The model under review builds one solid part; all positions refer to its coordinate system, in mm. Round coordinates to 2 decimals unless told otherwise and drop trailing zeros.
```python
from build123d import *

# Parameters (mm, degrees)
BOSS_EXTRUDE1_DEPTH   = 4.7625
M3_CLEARANCE_HOLE1_D  = 3.4
F_8_CLEARANCE_HOLE1_D = 4.4958
CIRPATTERN1_COUNT     = 12
CUT_EXTRUDE1_REACH    = 272.048
SKETCH15_W            = 6.35
SKETCH15_H            = 62.484
SKETCH15_W_2          = 5.116657908
SKETCH15_H_2          = 18.000886741
SKETCH15_H_3          = 20.68418835
SKETCH15_W_3          = 7.62
CUT_EXTRUDE2_REACH    = 272.048
SKETCH17_R            = 2.2479


with BuildPart() as part:
    # Sketch1 → Boss-Extrude1 (new body)
    with BuildSketch(Plane(origin=(0, 0, 0), x_dir=(1, 0, 0), z_dir=(0, 1, 0))):
        with BuildLine():
            Line((177.8, 98.373776994), (177.8, -98.373776994))
            ThreePointArc((177.8, -98.373776994), (0, -203.2), (-177.8, -98.373776994))
            Line((-177.8, -98.373776994), (-177.8, 98.373776994))
            ThreePointArc((-177.8, 98.373776994), (0, 203.2), (177.8, 98.373776994))
        make_face()
    extrude(amount=BOSS_EXTRUDE1_DEPTH)

    # M3 Clearance Hole1 (through all)
    with Locations(Plane(origin=(0, 4.7625, 0), x_dir=(1, 0, 0), z_dir=(0, 1, 0))):
        with Locations((174.55, -94.8), (174.55, -80), (174.55, -65.2), (174.55, 65.2), (174.55, 80), (174.55, 94.8)):
            m3_clearance_hole1 = Hole(M3_CLEARANCE_HOLE1_D / 2)

    # Mirror1: M3 Clearance Hole1 across plane
    add(m3_clearance_hole1.mirror(Plane(origin=(0, 0, 0), x_dir=(0, 0, 1), z_dir=(1, 0, 0))), mode=Mode.SUBTRACT)

    # #8 Clearance Hole1 (through all)
    with Locations(Plane(origin=(0, 4.7625, 0), x_dir=(1, 0, 0), z_dir=(0, 1, 0))):
        with Locations((0, -142.875)):
            f_8_clearance_hole1 = Hole(F_8_CLEARANCE_HOLE1_D / 2)

    # CirPattern1: #8 Clearance Hole1 ×12 about axis
    cirpattern1_axis = Axis((0, 0, 0), (0, 1, 0))
    for i in range(1, CIRPATTERN1_COUNT):
        add(f_8_clearance_hole1.rotate(cirpattern1_axis, i * 360 / CIRPATTERN1_COUNT), mode=Mode.SUBTRACT)

    # Sketch15 → Cut-Extrude1 (cut, up to next)
    with BuildSketch(Plane(origin=(0, 4.7625, 0), x_dir=(1, 0, 0), z_dir=(0, 1, 0)), mode=Mode.PRIVATE) as cut_extrude1_sk1:
        with Locations((24.765, 31.242)):
            Rectangle(SKETCH15_W, SKETCH15_H)
    cut_extrude1_tool1 = extrude(cut_extrude1_sk1.sketch, amount=-CUT_EXTRUDE1_REACH, mode=Mode.PRIVATE) & part.part
    # Sketch15 → Cut-Extrude1 (cut, up to next)
    with BuildSketch(Plane(origin=(0, 4.7625, 0), x_dir=(1, 0, 0), z_dir=(0, 1, 0)), mode=Mode.PRIVATE) as cut_extrude1_sk2:
        Polygon((-26.67, 62.484), (-33.02, 62.484), (-33.02, 60.402879746), (-40.64, 60.402879746), (-40.64, 42.401993005), (-33.02, 42.401993005), (-33.02, 0), (-26.67, 0), align=None)
    cut_extrude1_tool2 = extrude(cut_extrude1_sk2.sketch, amount=-CUT_EXTRUDE1_REACH, mode=Mode.PRIVATE) & part.part
    # Sketch15 → Cut-Extrude1 (cut, up to next)
    with BuildSketch(Plane(origin=(0, 4.7625, 0), x_dir=(1, 0, 0), z_dir=(0, 1, 0)), mode=Mode.PRIVATE) as cut_extrude1_sk3:
        with Locations((98.3234, 31.242)):
            Rectangle(SKETCH15_W, SKETCH15_H)
    cut_extrude1_tool3 = extrude(cut_extrude1_sk3.sketch, amount=-CUT_EXTRUDE1_REACH, mode=Mode.PRIVATE) & part.part
    # Sketch15 → Cut-Extrude1 (cut, up to next)
    with BuildSketch(Plane(origin=(0, 4.7625, 0), x_dir=(1, 0, 0), z_dir=(0, 1, 0)), mode=Mode.PRIVATE) as cut_extrude1_sk4:
        with Locations((-84.198328954, 51.402436376)):
            Rectangle(SKETCH15_W_2, SKETCH15_H_2)
    cut_extrude1_tool4 = extrude(cut_extrude1_sk4.sketch, amount=-CUT_EXTRUDE1_REACH, mode=Mode.PRIVATE) & part.part
    # Sketch15 → Cut-Extrude1 (cut, up to next)
    with BuildSketch(Plane(origin=(0, 4.7625, 0), x_dir=(1, 0, 0), z_dir=(0, 1, 0)), mode=Mode.PRIVATE) as cut_extrude1_sk5:
        with Locations((-84.198328954, -56.013830848)):
            Rectangle(SKETCH15_W_2, SKETCH15_H_3)
    cut_extrude1_tool5 = extrude(cut_extrude1_sk5.sketch, amount=-CUT_EXTRUDE1_REACH, mode=Mode.PRIVATE) & part.part
    # Sketch15 → Cut-Extrude1 (cut, up to next)
    with BuildSketch(Plane(origin=(0, 4.7625, 0), x_dir=(1, 0, 0), z_dir=(0, 1, 0)), mode=Mode.PRIVATE) as cut_extrude1_sk6:
        with Locations((-36.83, -56.013830848)):
            Rectangle(SKETCH15_W_3, SKETCH15_H_3)
    cut_extrude1_tool6 = extrude(cut_extrude1_sk6.sketch, amount=-CUT_EXTRUDE1_REACH, mode=Mode.PRIVATE) & part.part
    add(cut_extrude1_tool1.solids().sort_by_distance((24.765, 4.7625, -31.242))[0], mode=Mode.SUBTRACT)
    add(cut_extrude1_tool2.solids().sort_by_distance((-31.639414, 4.7625, -36.421123))[0], mode=Mode.SUBTRACT)
    add(cut_extrude1_tool3.solids().sort_by_distance((98.3234, 4.7625, -31.242))[0], mode=Mode.SUBTRACT)
    add(cut_extrude1_tool4.solids().sort_by_distance((-84.198329, 4.7625, -51.402436))[0], mode=Mode.SUBTRACT)
    add(cut_extrude1_tool5.solids().sort_by_distance((-84.198329, 4.7625, 56.013831))[0], mode=Mode.SUBTRACT)
    add(cut_extrude1_tool6.solids().sort_by_distance((-36.83, 4.7625, 56.013831))[0], mode=Mode.SUBTRACT)

    # Sketch17 → Cut-Extrude2 (cut, up to next)
    with BuildSketch(Plane(origin=(0, 4.7625, 0), x_dir=(1, 0, 0), z_dir=(0, 1, 0)), mode=Mode.PRIVATE) as cut_extrude2_sk1:
        with Locations(Location((40.402766773, 80.728472273, 0), (0, 0, 270))):
            Circle(SKETCH17_R)
    cut_extrude2_tool1 = extrude(cut_extrude2_sk1.sketch, amount=-CUT_EXTRUDE2_REACH, mode=Mode.PRIVATE) & part.part
    # Sketch17 → Cut-Extrude2 (cut, up to next)
    with BuildSketch(Plane(origin=(0, 4.7625, 0), x_dir=(1, 0, 0), z_dir=(0, 1, 0)), mode=Mode.PRIVATE) as cut_extrude2_sk2:
        with Locations(Location((9.538335251, -23.376368086, 0), (0, 0, 270))):
            Circle(SKETCH17_R)
    cut_extrude2_tool2 = extrude(cut_extrude2_sk2.sketch, amount=-CUT_EXTRUDE2_REACH, mode=Mode.PRIVATE) & part.part
    add(cut_extrude2_tool1.solids().sort_by_distance((40.402767, 4.7625, -80.728472))[0], mode=Mode.SUBTRACT)
    add(cut_extrude2_tool2.solids().sort_by_distance((9.538335, 4.7625, 23.376368))[0], mode=Mode.SUBTRACT)


solid = part.part
```
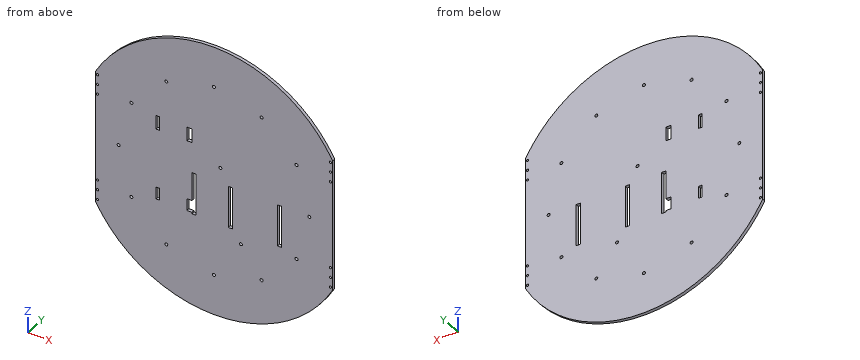
(1) Consider section A-A (y = 1). State how many separate pieces and enclosed holes the cut face has, and give its area (3 significant figures).
Data:
separate pieces: 1
enclosed holes: 32
area: 121,000 mm2
(2) To check wall thickness, follow probe 1 along X at (y, z) = (3.5, -4); probe 2 along X at (y, z) = (1.1, 47); probe 3 along X at (y, z) = (1.45, -60). State the ranges of each line that lie inside material, in increasing order.
Data:
probe 1: x = -177.8 to -33.02, -26.67 to 21.59, 27.94 to 95.15, 101.5 to 177.8
probe 2: x = -177.8 to -86.76, -81.64 to -40.64, -33.02 to 177.8
probe 3: x = -177.8 to -86.76, -81.64 to -40.64, -26.67 to 21.59, 27.94 to 95.15, 101.5 to 177.8
(3) Insertion check: pin 1 (4 mm diameter, centred on x = 71.44, z = -123.73, fed in from -Y); pin 2 (2.5 mm diameter, centred on x = -30.5, y = 2.5, fed in from -Z). Each pin has a flat end and moves straight along its axis. Give the tip position at first contact, or say it passes through.
Data:
pin 1: passes through
pin 2: stops at z = -201.08
